Check sheet for the modelled part. Datum: model origin and axes. Units: mm. Face numbers are marked on the shaded views. A direction names the side the tool comes from. Give positions to 0.01 mm unless a question says otherwise; leave off trailing zeros. Write each loop counter-clockwise with the first axis right and the second up, starting at its lowest first coordinate (ties: lowest second). Pieces come first, ordered by that corner, then holes. Notation, with made-up numbers: (-1, -6) -> (32, -6) arc R21 ccw to (32, 2) -> close; hole circle Ø5 at (21.25, -8.75). An arc over 180 degrees is marked (long way). Use a Markdown table: item, result. Add a question column.
1. Set-up check for the marked faces 1 and 2: record each of +Z, -Z, +X, -X, +Y, -Y from which the full face is reachable in a straight line by a thin tool's end or side.
2. Cross-section at A-A (x = -35). Enter the section's corners in (y, z).
3. Cross-section at B-B (y = 32.5). Enter the section's corners in (x, z).
4. Cross-section at D-D (z = -3). Enter the section's corners in (x, y).
5. Scan lines: probe 1 along Y at (x, z) = (-47.5, -4.25); probe 2 along X at (y, z) = (19.5, -1); probe 3 along Y at (x, z) = (-35, -2.75). Record each from-to range of solid material in increasing order. Write a range as [from, to].
6. Cross-section at C-C (x = -47.5). Enter the section's corners in (y, z), then the cut area to 3 significant figures.
7. Release check for a two-part mould opening along X. For the marked faces 3, 4 and 5 record: released by +X, released by -X, zero draft, split by the parting line, or undercut.
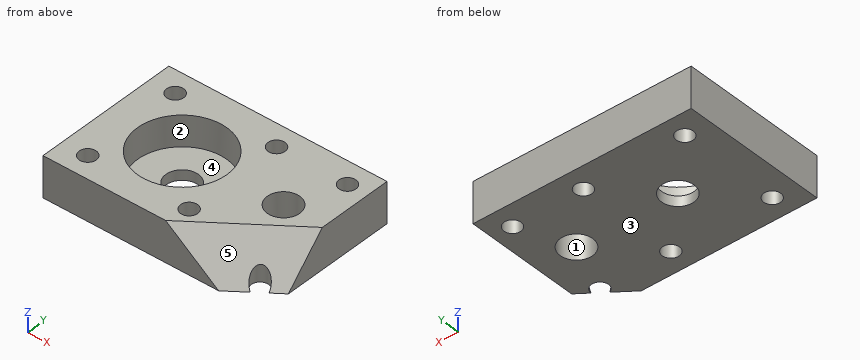
from build123d import *

# Parameters (mm, degrees)
JOTYY_MIRRORED_START         = -10
JOTYY_MIRRORED_OUTLINE_W     = 53.8
JOTYY_MIRRORED_OUTLINE_H     = 36
JOTYY_MIRRORED_OUTLINE_R     = 2.1
JOTYY_MIRRORED_OUTLINE_R_2   = 11
JOTYY_MIRRORED_DEPTH         = 10
JOTYY_MIRRORED_2_OUTLINE_R   = 11
JOTYY_MIRRORED_2_OUTLINE_R_2 = 4
JOTYY_MIRRORED_2_DEPTH       = 2.5
SKETCH1_R                    = 4
CUT_EXTRUDE1_DEPTH           = 10
CUT_EXTRUDE2_DEPTH           = 58.211226571


# Read off the part's stored shape, not the designer's step: jotyy_Mirrored
with BuildPart() as part:
    # jotyy_Mirrored outline → jotyy_Mirrored (new body)
    with BuildSketch(Plane.XY.offset(JOTYY_MIRRORED_START)):
        with Locations((-26.9, 20)):
            Rectangle(JOTYY_MIRRORED_OUTLINE_W, JOTYY_MIRRORED_OUTLINE_H)
        with Locations((-47.5, 7.5)):
            Circle(JOTYY_MIRRORED_OUTLINE_R, mode=Mode.SUBTRACT)
        with Locations((-22.5, 7.5)):
            Circle(JOTYY_MIRRORED_OUTLINE_R, mode=Mode.SUBTRACT)
        with Locations((-5, 7.5)):
            Circle(JOTYY_MIRRORED_OUTLINE_R, mode=Mode.SUBTRACT)
        with Locations((-35, 20)):
            Circle(JOTYY_MIRRORED_OUTLINE_R_2, mode=Mode.SUBTRACT)
        with Locations((-47.5, 32.5)):
            Circle(JOTYY_MIRRORED_OUTLINE_R, mode=Mode.SUBTRACT)
        with Locations((-22.5, 32.5)):
            Circle(JOTYY_MIRRORED_OUTLINE_R, mode=Mode.SUBTRACT)
        with Locations((-5, 32.5)):
            Circle(JOTYY_MIRRORED_OUTLINE_R, mode=Mode.SUBTRACT)
    extrude(amount=JOTYY_MIRRORED_DEPTH)

    # jotyy_Mirrored 2 outline → jotyy_Mirrored 2 (add)
    with BuildSketch(Plane.XY.offset(JOTYY_MIRRORED_START)):
        with Locations((-35, 20)):
            Circle(JOTYY_MIRRORED_2_OUTLINE_R)
        with Locations((-35, 20)):
            Circle(JOTYY_MIRRORED_2_OUTLINE_R_2, mode=Mode.SUBTRACT)
    extrude(amount=JOTYY_MIRRORED_2_DEPTH)

    # Sketch1 → Cut-Extrude1 (cut)
    with BuildSketch(Plane.XY):
        with Locations((-10, 20)):
            Circle(SKETCH1_R)
    extrude(amount=-CUT_EXTRUDE1_DEPTH, mode=Mode.SUBTRACT)

    # Sketch4 → Cut-Extrude2 (cut, through all)
    with BuildSketch(Plane(origin=(-5.803979924, 7.804579549, -7.598887182), x_dir=(-0.8814294563143725, -0.3015166465944173, 0.36355168183878195), z_dir=(-0.47023817530075585, 0.6323266610618664, -0.6156614753256593))):
        Polygon((64.66091517, 41.829227813), (-62.885997207, -203.452641014), (-179.111332111, -143.015305479), (-51.564419733, 102.266563348), align=None)
    extrude(amount=-CUT_EXTRUDE2_DEPTH, mode=Mode.SUBTRACT)


solid = part.part
Worked answers:
| question | item | result |
|---|---|---|
| 1 | face 1 | +Z, -Z |
| 1 | face 2 | +Z |
| 2 | outline | (2, -10) -> (16, -10) -> (16, -7.5) -> (9, -7.5) -> (9, 0) -> (2, 0) -> close; (24, -10) -> (38, -10) -> (38, 0) -> (31, 0) -> (31, -7.5) -> (24, -7.5) -> close |
| 3 | outline | (-53.8, -10) -> (-49.6, -10) -> (-49.6, 0) -> (-53.8, 0) -> close; (-45.4, -10) -> (-24.6, -10) -> (-24.6, 0) -> (-45.4, 0) -> close; (-20.4, -10) -> (-7.1, -10) -> (-7.1, 0) -> (-20.4, 0) -> close; (-2.9, -10) -> (0, -10) -> (0, 0) -> (-2.9, 0) -> close |
| 4 | outline | (-53.8, 2) -> (-19.63, 2) -> (0, 16.6) -> (0, 38) -> (-53.8, 38) -> close; hole circle Ø4.2 at (-47.5, 7.5); hole circle Ø4.2 at (-47.5, 32.5); hole circle Ø22 at (-35, 20); hole circle Ø4.2 at (-22.5, 7.5); hole circle Ø4.2 at (-22.5, 32.5); hole circle Ø8 at (-10, 20); hole circle Ø4.2 at (-5, 32.5) |
| 5 | probe 1 | y = [2, 5.4], [9.6, 30.4], [34.6, 38] |
| 5 | probe 2 | x = [-53.8, -45.99], [-24.01, -13.97], [-6.03, 0] |
| 5 | probe 3 | y = [2, 9], [31, 38] |
| 6 | outline | (2, -10) -> (5.4, -10) -> (5.4, 0) -> (2, 0) -> close; (9.6, -10) -> (30.4, -10) -> (30.4, 0) -> (9.6, 0) -> close; (34.6, -10) -> (38, -10) -> (38, 0) -> (34.6, 0) -> close |
| 6 | area | 276 mm² |
| 7 | face 3 | zero draft |
| 7 | face 4 | undercut |
| 7 | face 5 | released by +X |
